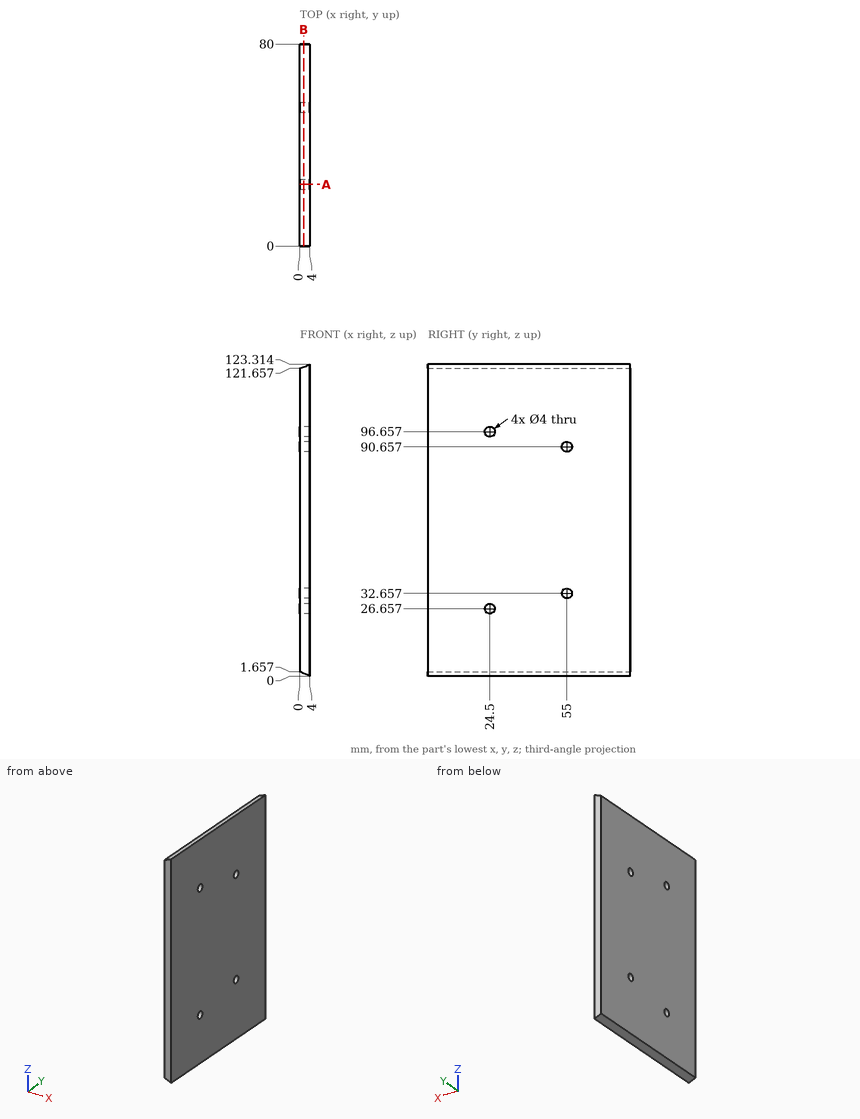
Here's the drawing with two shaded views (mm, measured from the low corner). I have some questions. Round coordinates to 2 decimals unless told otherwise and drop trailing zeros. Loops run counter-clockwise (first coordinate to the right, second up) from the corner with the lowest first, then second, coordinate; pieces in that order, holes last. Notation, with made-up numbers: (-14.75, 29.5) -> (7.25, 29.5) arc R37 ccw to (7.25, 65.5) -> close; hole circle Ø11 at (81, 12). An arc over 180 degrees is marked (long way). Answer as CSV lines item,"result". Start each with the question number.
1. Imagine slicing it at A-A on y = 24.5. Write out the boundary of the cut face in (x, z).
2. Imagine slicing it at B-B on x = 1.5. Write out the boundary of the cut face in (y, z) (1 decimal).
3. I'm going to push flat-ended pins straight in: P1, Ø1, axis at x = 1, y = 58.5, coming from the +Z side; P2, Ø3, axis at y = 24.5, z = 26.66, coming from the -X side; P3, Ø1, axis at x = 2.5, y = 57, coming from the +Z side. Where does each tip first touch, or does it pass through?
4. I need wall thicknesses on probe 1 along Z at (x, y) = (2.65, 24.5) (1 decimal); probe 2 along Y at (x, z) = (1.7, 90.5); probe 3 along Z at (x, y) = (2.85, 24.5). Which ranges of each line are inside material? Lowest first, please. Write a range as from..to.
Solution:
1,outline,"(0, 1.66) -> (4, 0) -> (4, 24.66) -> (0, 24.66) -> close; (0, 28.66) -> (4, 28.66) -> (4, 94.66) -> (0, 94.66) -> close; (0, 98.66) -> (4, 98.66) -> (4, 123.31) -> (0, 121.66) -> close"
2,outline,"(0, 1) -> (80, 1) -> (80, 122.3) -> (0, 122.3) -> close; hole circle Ø4 at (24.5, 26.7); hole circle Ø4 at (24.5, 96.7); hole circle Ø4 at (55, 32.7); hole circle Ø4 at (55, 90.7)"
3,P1,"z = 122.28"
3,P2,"through"
3,P3,"z = 122.9"
4,probe 1,"0.6..24.7, 28.7..94.7, 98.7..122.8"
4,probe 2,"0..53.01, 56.99..80"
4,probe 3,"0.48..24.66, 28.66..94.66, 98.66..122.84"
